Design review of the part built by this model. Coordinates are the model's own, in mm. A direction names the side the tool comes from. Give positions to 0.01 mm unless a question says otherwise; leave off trailing zeros. Order: outer loops, then holes, each group sorted by start corner. A loop starts at its lowest first (then second) coordinate and runs counter-clockwise, first axis right, second up. Notation, with made-up numbers: M -23,-23.5 L -15,-23.5 A29 cw -15,8.5 Z; hole C 18,84.25 d6. An arc over 180 degrees is marked long. Answer as a JSON object with one key per item and string values.
from build123d import *

# Parameters (mm, degrees)
SKETCH_1_R          = 3.75
EXTRUDE_2_DEPTH     = 1.6
SKETCH_2_R          = 1.5
CUT_EXTRUDE_1_DEPTH = 2
SKETCH_3_R          = 2.75
EXTRUDE_3_DEPTH     = 0.5
SKETCH_4_R          = 1.5
CUT_EXTRUDE_2_DEPTH = 3
FILLET_1_R          = 0.1


with BuildPart() as part:
    # 草图1 → 凸台-拉伸2 (new body)
    with BuildSketch(Plane(origin=(0, 0, 0), x_dir=(1, 0, 0), z_dir=(0, 1, 0))):
        with Locations(Location((0, 0, 0), (0, 0, 270))):
            Circle(SKETCH_1_R)
    extrude(amount=EXTRUDE_2_DEPTH)

    # 草图2 → 切除-拉伸1 (cut)
    with BuildSketch(Plane(origin=(0, 1.6, 0), x_dir=(1, 0, 0), z_dir=(0, 1, 0))):
        with Locations(Location((0, 0, 0), (0, 0, 270))):
            Circle(SKETCH_2_R)
    extrude(amount=-CUT_EXTRUDE_1_DEPTH, mode=Mode.SUBTRACT)

    # 草图3 → 凸台-拉伸3 (add)
    with BuildSketch(Plane(origin=(0, 1.6, 0), x_dir=(1, 0, 0), z_dir=(0, 1, 0))):
        with Locations(Location((0, 0, 0), (0, 0, 270))):
            Circle(SKETCH_3_R)
    extrude(amount=EXTRUDE_3_DEPTH)

    # 草图4 → 切除-拉伸2 (cut)
    with BuildSketch(Plane(origin=(0, 2.1, 0), x_dir=(1, 0, 0), z_dir=(0, 1, 0))):
        with Locations(Location((0, 0, 0), (0, 0, 270))):
            Circle(SKETCH_4_R)
    extrude(amount=-CUT_EXTRUDE_2_DEPTH, mode=Mode.SUBTRACT)

    # 圆角1
    fillet_1_edges = [part.edges().sort_by_distance(p)[0] for p in [
        (0, 2.1, -2.75),
        (0, 2.1, -1.5),
        (0, 0, -3.75),
        (0, 1.6, -3.75),
        (0, 0, -1.5),
    ]]
    fillet(fillet_1_edges, radius=FILLET_1_R)


solid = part.part
(1) Draft analysis for pull direction Z (two halves, no side actions). For faces 3 (the cylindrical face through (0.45, 1.06, 1.43)), 4 (the cylindrical face through (0.165, 0.79, -3.746)), 5 (the flat face through (-2, 0, 1)), state which applies: +Z half, -Z half, draft (parallel to the pull), parting line (faces both ways), or undercut.
Checked values:
{"face 3": "undercut", "face 4": "parting line", "face 5": "draft"}
(2) We need section C-C (y = 1.4). Write out the cut boundary in (x, z), plus the area to 3 significant figures.
Checked values:
{"outline": "C 0,0 d7.5; hole C 0,0 d3", "area": "37.1 mm^2"}
(3) Tool access review of faces 1 (the cylindrical face through (-2.685, 1.797, -0.596)), 2 (the flat face through (0, 2.1, 2)): name each direction out of +Z, -Z, +X, -X, +Y, -Y from which nothing blocks a thin tool from reaching the whole face with its end or side.
Checked values:
{"face 1": "+Y", "face 2": "+Z, -Z, +X, -X, +Y"}
(4) We need section D-D (y = 1.8). Write out the cut boundary in (x, z), plus the area to 3 significant figures.
Checked values:
{"outline": "C 0,0 d5.5; hole C 0,0 d3", "area": "16.7 mm^2"}
(5) We need section B-B (z = 0). Write out the cut boundary in (x, y).
Checked values:
{"outline": "M -3.75,0.1 A0.1 ccw -3.65,0 L -1.6,0 A0.1 ccw -1.5,0.1 L -1.5,2 A0.1 ccw -1.6,2.1 L -2.65,2.1 A0.1 ccw -2.75,2 L -2.75,1.6 L -3.65,1.6 A0.1 ccw -3.75,1.5 Z; M 1.5,0.1 A0.1 ccw 1.6,0 L 3.65,0 A0.1 ccw 3.75,0.1 L 3.75,1.5 A0.1 ccw 3.65,1.6 L 2.75,1.6 L 2.75,2 A0.1 ccw 2.65,2.1 L 1.6,2.1 A0.1 ccw 1.5,2 Z"}
(6) To check wall thickness, follow L1, parallel to X at y = 0.35, z = 0; L2, parallel to Y at x = -2, z = 2.25; L3, parallel to Z at x = 1.25, y = 1.1. State the ranges of each line that lie inside material, in increasing order. Write a range as from..to.
Checked values:
{"L1": "x = -3.75..-1.5, 1.5..3.75", "L2": "y = 0..1.6", "L3": "z = -3.54..-0.83, 0.83..3.54"}
(7) Insertion check: pin 1 (2.5 mm diameter, centred on x = 0, z = 0, fed in from +Y); pin 2 (4 mm diameter, centred on x = -1, z = -1.5, fed in from -Y). Each pin has a flat end and moves straight along its axis. Give the tip position at first contact, or say it passes through.
Checked values:
{"pin 1": "passes through", "pin 2": "stops at y = 0"}
(8) We need section A-A (x = 0). Write out the cut boundary in (y, z).
Checked values:
{"outline": "M 0,-3.65 A0.1 ccw 0.1,-3.75 L 1.5,-3.75 A0.1 ccw 1.6,-3.65 L 1.6,-2.75 L 2,-2.75 A0.1 ccw 2.1,-2.65 L 2.1,-1.6 A0.1 ccw 2,-1.5 L 0.1,-1.5 A0.1 ccw 0,-1.6 Z; M 0,1.6 A0.1 ccw 0.1,1.5 L 2,1.5 A0.1 ccw 2.1,1.6 L 2.1,2.65 A0.1 ccw 2,2.75 L 1.6,2.75 L 1.6,3.65 A0.1 ccw 1.5,3.75 L 0.1,3.75 A0.1 ccw 0,3.65 Z"}
